CAD build for the part. Positions are in the model's coordinates, mm. A direction names the side the tool comes from. Give positions to 0.01 mm unless a question says otherwise; leave off trailing zeros. Write each loop counter-clockwise with the first axis right and the second up, starting at its lowest first coordinate (ties: lowest second). Pieces come first, ordered by that corner, then holes. Notation, with made-up numbers: (-10, 8.25) - (37, 8.25) arc R23 ccw to (37, 32.25) - close; hole circle Ø9 at (87, 82.25). An arc over 180 degrees is marked (long way). Put each result on its own line as item: value. Start each with the question number.
1. Wall check: line 1 (X direction, y = -2.4, z = 28.25); line 2 (Y direction, x = -27, z = 30.5); line 3 (Z direction, x = -24.25, y = -1.05). Give the ranges that are in metal, low to high.
2. Cut at C-C on x = -22. List the corners of the cut face in (y, z).
3. Tool access for faces 1 (the flat face through (-22.933, -2, 29)), 2 (the flat face through (-25, -3.2, 29)), 3 (the flat face through (-27.642, -2, 29)), 4 (the flat face through (-25, -1.5, 29)): list every direction of +Z, -Z, +X, -X, +Y, -Y with a clear straight run to the whole face (end or side of a thin tool).
4. Cut at B-B on z = 42.5. List the corners of the cut face in (x, y).
5. Drop flat-ended pins along their axis: pin 1 (1.5 mm diameter, centred on x = -22.5, z = 43.5, fed in from +Y); pin 2 (1.4 mm diameter, centred on y = -2, z = 29.5, fed in from -X); pin 3 (1 mm diameter, centred on y = -1.5, z = 31, fed in from +X); pin 4 (4 mm diameter, centred on x = -26, z = 29, fed in from +Y). Give the stop position or say it passes through.
6. Cut at A-A on y = -1.75. List the corners of the cut face in (x, z).
7. Cut at D-D on y = -4.15. List the corners of the cut face in (x, z).
from build123d import *

# Parameters (mm, degrees)
F0_W     = 7.7586211264
F0_H     = 13.5775841773
F1_DEPTH = 4.7
F2_DEPTH = 0.05
F3_R     = 1.5
F4_DEPTH = 5.34


with BuildPart() as f1:
    # F0 (on Front) → F1 (new body)
    with BuildSketch(Plane.XZ):
        with Locations((-25.3125019372, 38.5021548718)):
            Rectangle(F0_W, F0_H)
    extrude(amount=F1_DEPTH)

    # F2 (cut): a face of the model
    f2_faces = [f1.faces().sort_by_distance(p)[0] for p in [
        (-29.1918125004, -2.35, 38.5021548718),
    ]]
    extrude(f2_faces, amount=-F2_DEPTH, mode=Mode.SUBTRACT)

    # F3
    f3_edges = [f1.edges().sort_by_distance(p)[0] for p in [
        (-29.141813, -4.7, 38.502155),
        (-29.141813, 0, 38.502155),
        (-21.433191, 0, 38.502155),
        (-21.433191, -4.7, 38.502155),
        (-25.287502, -4.7, 31.713363),
        (-25.287502, 0, 31.713363),
        (-21.433191, -2.35, 31.713363),
        (-29.141813, -2.35, 31.713363),
    ]]
    fillet(f3_edges, radius=F3_R)

    # F4 (add): a face of the model
    f4_faces = [f1.faces().sort_by_distance(p)[0] for p in [
        (-25.2875019372, -2.35, 31.7133627832),
    ]]
    extrude(f4_faces, amount=F4_DEPTH)


solid = f1.part
Report:
1. line 1: x = -27.64 to -22.93
1. line 2: y = -3.2 to -1.5
1. line 3: z = 31.78 to 45.29
2. outline: (-4.37, 33.21) arc R1.17 ccw to (-3.2, 32.04) - (-1.5, 32.04) arc R1.17 ccw to (-0.33, 33.21) - (-0.33, 45.29) - (-4.37, 45.29) - close
3. face 1: -Z, +X, +Y, -Y
3. face 2: -Z, +X, -X, -Y
3. face 3: -Z, -X, +Y, -Y
3. face 4: -Z, +X, -X, +Y
4. outline: (-29.14, -3.2) arc R1.5 ccw to (-27.64, -4.7) - (-22.93, -4.7) arc R1.5 ccw to (-21.43, -3.2) - (-21.43, -1.5) arc R1.5 ccw to (-22.93, 0) - (-27.64, 0) arc R1.5 ccw to (-29.14, -1.5) - close
5. pin 1: stops at y = 0
5. pin 2: stops at x = -27.64
5. pin 3: stops at x = -22.93
5. pin 4: stops at y = -1.5
6. outline: (-29.14, 33.21) arc R1.5 ccw to (-27.64, 31.71) - (-27.64, 26.37) - (-22.93, 26.37) - (-22.93, 31.71) arc R1.5 ccw to (-21.43, 33.21) - (-21.43, 45.29) - (-29.14, 45.29) - close
7. outline: (-28.8, 33.21) arc R1.16 ccw to (-27.64, 32.05) - (-22.93, 32.05) arc R1.16 ccw to (-21.77, 33.21) - (-21.77, 45.29) - (-28.8, 45.29) - close
